```python
from build123d import *

# Parameters (mm, degrees)
F0_W     = 100
F0_H     = 50
F1_DEPTH = 20
F2_W     = 45
F2_H     = 50
F3_DEPTH = 50
F4_W     = 25
F4_H     = 60
F5_DEPTH = 50.001
F6_R     = 10
F7_DEPTH = 45
F8_R     = 7.5
F9_DEPTH = 10
F10_R    = 1
F11_SIZE = 1


with BuildPart() as f1:
    # F0 (on Top) → F1 (new body)
    with BuildSketch(Plane.XY):
        with Locations((50, 25)):
            Rectangle(F0_W, F0_H)
    extrude(amount=F1_DEPTH)

    # F2 (on face) → F3 (join)
    with BuildSketch(Plane.XY.offset(20)):
        with Locations((22.5, 25)):
            Rectangle(F2_W, F2_H)
    extrude(amount=F3_DEPTH)

    # F4 (on face) → F5 (cut, through all)
    with BuildSketch(Plane.XZ):
        with Locations((22.5, 30)):
            Rectangle(F4_W, F4_H)
    extrude(amount=-F5_DEPTH, mode=Mode.SUBTRACT)

    # F6 (on face) → F7 (cut, through all)
    with BuildSketch(Plane(origin=(0, 0, 0), x_dir=(0, -1, 0), z_dir=(-1, 0, 0))):
        with Locations((-25, 40)):
            Circle(F6_R)
    extrude(amount=-F7_DEPTH, mode=Mode.SUBTRACT)

    # F8 (on face) → F9 (cut, through all)
    with BuildSketch(Plane.XY.offset(70)):
        with Locations((22.5, 25)):
            Circle(F8_R)
    extrude(amount=-F9_DEPTH, mode=Mode.SUBTRACT)

    # F10
    f10_edges = [f1.edges().sort_by_distance(p)[0] for p in [
        (45, 25, 70),
        (45, 25, 20),
        (45, 0, 45),
        (22.5, 0, 70),
        (0, 0, 35),
        (0, 25, 70),
        (22.5, 50, 70),
        (45, 50, 45),
        (72.5, 50, 20),
        (100, 25, 20),
        (0, 50, 35),
        (100, 0, 10),
        (100, 50, 10),
        (72.5, 0, 20),
    ]]
    fillet(f10_edges, radius=F10_R)

    # F11
    f11_edges = [f1.edges().sort_by_distance(p)[0] for p in [
        (45, 35, 40),
        (10, 35, 40),
        (35, 35, 40),
        (0, 35, 40),
        (15, 25, 70),
        (15, 25, 60),
    ]]
    chamfer(f11_edges, length=F11_SIZE)


solid = f1.part
```
Source: CAD feature listing. Evaluate the final solid. Frame: model axes, mm. A direction names the side the tool comes from. Round coordinates to 2 decimals unless told otherwise and drop trailing zeros. Write each loop counter-clockwise with the first axis right and the second up, starting at its lowest first coordinate (ties: lowest second). Pieces come first, ordered by that corner, then holes. Notation, with made-up numbers: M -31.75,1 L -22.75,1 A27 cw -22.75,39 Z; hole C 30.5,9 d10. An arc over 180 degrees is marked long. Answer as a JSON object with one key per item and string values. Group by question number.
(1) Section query A-A on z = 12.5. Output: boundary loops of the cut face in (x, y).
(2) First-contact query: pin 1 (2 mm diameter, centred on y = 18.5, z = 51, fed in from -X); pin 2 (1.5 mm diameter, centred on x = 87.5, y = 5.5, fed in from +Z); pin 3 (1 mm diameter, centred on y = 29.5, z = 50, fed in from +X); pin 4 (18 mm diameter, centred on y = 25, z = 40, fed in from +X). Flat tips, straight axial feed; report the tip coordinate or a pass-through.
(3) Mould query, pull axis Y, two halves, no side actions, for faces 1 (the flat face through (35, 25, 23)), 2 (the flat face through (38, 0, 26)), 3 (the cylindrical face through (4.944, 20.386, 31.128)), 4 (the flat face through (38, 50, 26)). Classes: +Y half, -Y half, draft (parallel to the pull), parting line (faces both ways), or undercut.
(4) Section query C-C on x = 22.5. Output: boundary loops of the cut face in (y, z).
(5) Reachability of faces 5 (the flat face through (14, 19, 60)), 6 (the flat face through (67, 25, 0)), 7 (the flat face through (72, 25, 20)) from +Z, -Z, +X, -X, +Y, -Y: full face, straight path, thin tool, end or side. Return the list, or none.
(6) Ray query, line 1 (X direction, y = 7.5, z = 11.5); line 2 (X direction, y = 39.5, z = 45); line 3 (Y direction, x = 22, z = 67). Return the intervals inside material, ascending. Write a range as [from, to].
(7) Section query D-D on y = 3.5. Output: boundary loops of the cut face in (x, z).
(8) Section query B-B on z = 40. Output: boundary loops of the cut face in (x, y).
Computed values:
{
 "1": {"outline": "M 0,1 A1 ccw 1,0 L 10,0 L 10,50 L 1,50 A1 ccw 0,49 Z; M 35,0 L 99,0 A1 ccw 100,1 L 100,49 A1 ccw 99,50 L 35,50 Z"},
 "2": {"pin 1": "x = 0", "pin 2": "z = 20", "pin 3": "x = 45", "pin 4": "through"},
 "3": {"face 1": "draft", "face 2": "-Y half", "face 3": "undercut", "face 4": "+Y half"},
 "4": {"outline": "M 0,60 L 16.5,60 L 17.5,61 L 17.5,69 L 16.5,70 L 1,70 A1 ccw 0,69 Z; M 32.5,61 L 33.5,60 L 50,60 L 50,69 A1 ccw 49,70 L 33.5,70 L 32.5,69 Z"},
 "5": {"face 5": "-Z, +Y, -Y", "face 6": "-Z, +X, -X, +Y, -Y", "face 7": "+Z, +X, +Y, -Y"},
 "6": {"line 1": "[0, 10], [35, 100]", "line 2": "[0, 10], [35, 45]", "line 3": "[0, 17.52], [32.48, 50]"},
 "7": {"outline": "M 0,0 L 10,0 L 10,60 L 35,60 L 35,0 L 100,0 L 100,19 A1 ccw 99,20 L 46,20 A1 cw 45,21 L 45,69 A1 ccw 44,70 L 1,70 A1 ccw 0,69 Z"},
 "8": {"outline": "M 0,1 A1 ccw 1,0 L 10,0 L 10,14 L 9,15 L 1,15 L 0,14 Z; M 0,36 L 1,35 L 9,35 L 10,36 L 10,50 L 1,50 A1 ccw 0,49 Z; M 35,0 L 44,0 A1 ccw 45,1 L 45,14 L 44,15 L 36,15 L 35,14 Z; M 35,36 L 36,35 L 44,35 L 45,36 L 45,49 A1 ccw 44,50 L 35,50 Z"}
}
